Verification items for the finished model (mm, model axes). A direction names the side the tool comes from. Give positions to 0.01 mm unless a question says otherwise; leave off trailing zeros. Loops run counter-clockwise (first coordinate to the right, second up) from the corner with the lowest first, then second, coordinate; pieces in that order, holes last. Notation, with made-up numbers: (35.25, 86.5) -> (81.25, 86.5) arc R18 cw to (81.25, 92.5) -> close; hole circle Ø5 at (-7.5, -11). An arc over 180 degrees is marked (long way). Answer in a Markdown table with one row per item. Add a question column.
Q1. Gauge pin test, flat ends, axial feed: P1, Ø4, axis at x = 78.97, y = 68.18, coming from the +Z side; P2, Ø6, axis at y = 53, z = 3, coming from the +X side; P3, Ø6.5, axis at y = 95.5, z = 8, coming from the +X side; P4, Ø4, axis at x = 144, z = 3, coming from the -Y side. Record the tip position at first contact, or that the pin passes through.
Q2. Material ranges on probe 1 along Y at (x, z) = (88, 7.25); probe 2 along X at (y, z) = (67, 4.25); probe 3 along X at (y, z) = (43.5, 6), recorded low to high.
Q3. Section check B-B on z = 2.5. Give the number of separate pieces and of enclosed holes in the cut face, and give its area (3 significant figures).
Q4. Release check for a two-part mould opening along X. For faces 4 (the face through (6.16, 62, 6.41)), 5 (the face through (143.55, 20.69, 6.41)), 6 (the face through (38.49, 7.41, 6.41)) record: pulls with the +X half, pulls with the -X half, needs draft (parallel to the pull), parting line crosses it, or undercut.
Q5. Section check D-D on y = 36. Enter the section's corners in (x, z).
Q6. Section check A-A on y = 47. Enter the section's corners in (x, z).
Q7. Section check C-C on x = 153.5. Enter the section's corners in (y, z).
Q8. Set-up check for faces 1 (the face through (59.37, 14.43, 6.41)), 2 (the face through (128.62, 71.9, 6.41)), 3 (the face through (146.511, 82.857, 6.409)): record each of +Z, -Z, +X, -X, +Y, -Y from which the full face is reachable in a straight line by a thin tool's end or side.
```python
from build123d import *

# Parameters (mm, degrees)
ESBO_O1_R                = 3.175
RESSALTO_EXTRUS_O1_DEPTH = 13


with BuildPart() as part:
    # Esboço1 → Ressalto-extrusão1 (new body)
    with BuildSketch(Plane.XY):
        with BuildLine():
            Line((35.385230037, 10.075467345), (3.022965856, 59.821309359))
            Line((3.022965856, 59.821309359), (9.389592457, 64.241305524))
            ThreePointArc((9.389592457, 64.241305524), (12.424025355, 62.134521854), (16.11664555, 62.238812532))
            Line((16.11664555, 62.238812532), (37.995734983, 76.310625699))
            Line((37.995734983, 76.310625699), (73.510181395, 78.362700262))
            ThreePointArc((73.510181395, 78.362700262), (77.993066809, 80.699414035), (80.140456658, 85.276007717))
            Line((80.140456658, 85.276007717), (79.930003073, 94.415706286))
            Line((79.930003073, 94.415706286), (79.930003073, 97.029046835))
            ThreePointArc((79.930003073, 97.029046835), (101.572218687, 91.878964915), (121.946388489, 100.812163968))
            Line((121.946388489, 100.812163968), (121.946388489, 97.854479056))
            Line((121.946388489, 97.854479056), (121.946388489, 87.306940797))
            ThreePointArc((121.946388489, 87.306940797), (124.605004373, 83.87722317), (128.400566482, 81.773676237))
            Line((128.400566482, 81.773676237), (165.135958914, 83.971302002))
            Line((165.135958914, 83.971302002), (186.825026221, 73.136677472))
            ThreePointArc((186.825026221, 73.136677472), (191.417140339, 72.651683009), (195.305426608, 75.142458308))
            Line((195.305426608, 75.142458308), (201.904648359, 71.689614729))
            ThreePointArc((201.904648359, 71.689614729), (180.384547639, 42.366647273), (150.812504997, 21.190116644))
            ThreePointArc((150.812504997, 21.190116644), (150.313679981, 20.942400372), (149.813666262, 20.697092344))
            ThreePointArc((149.813666262, 20.697092344), (143.468376798, 20.722988132), (139.020600507, 25.248543905))
            ThreePointArc((139.020600507, 25.248543905), (106.562536674, 52.191838172), (72.546533139, 27.244322919))
            ThreePointArc((72.546533139, 27.244322919), (59.147798476, 14.281047119), (41.970794252, 7.033762392))
            ThreePointArc((41.970794252, 7.033762392), (38.439332559, 7.432489412), (35.662068876, 9.64992292))
            Line((35.662068876, 9.64992292), (35.385230037, 10.075467345))
        make_face()
        with Locations((89.421948725, 79.437523552)):
            Circle(ESBO_O1_R, mode=Mode.SUBTRACT)
        with Locations((113.572558486, 80.849829661)):
            Circle(ESBO_O1_R, mode=Mode.SUBTRACT)
        with Locations((78.965142383, 68.179773497)):
            Circle(ESBO_O1_R, mode=Mode.SUBTRACT)
        with Locations((125.590943677, 70.946640577)):
            Circle(ESBO_O1_R, mode=Mode.SUBTRACT)
    extrude(amount=RESSALTO_EXTRUS_O1_DEPTH)


solid = part.part
```
Taken from the geometry:
| question | item | result |
|---|---|---|
| 1 | P1 | passes through |
| 1 | P2 | stops at x = 192.18 |
| 1 | P3 | stops at x = 121.95 |
| 1 | P4 | stops at y = 20.1 |
| 2 | probe 1 | y = 47.38 to 76.6, 82.28 to 93.33 |
| 2 | probe 2 | x = 23.52 to 76.02, 81.91 to 199.35 |
| 2 | probe 3 | x = 13.64 to 82.71, 128.36 to 181.52 |
| 3 | separate pieces | 1 |
| 3 | enclosed holes | 4 |
| 3 | area | 8,820 mm² |
| 4 | face 4 | pulls with the -X half |
| 4 | face 5 | undercut |
| 4 | face 6 | parting line crosses it |
| 5 | outline | (18.52, 0) -> (76.41, 0) -> (76.41, 13) -> (18.52, 13) -> close; (134.66, 0) -> (173.39, 0) -> (173.39, 13) -> (134.66, 13) -> close |
| 6 | outline | (11.36, 0) -> (87.37, 0) -> (87.37, 13) -> (11.36, 13) -> close; (123.7, 0) -> (184.82, 0) -> (184.82, 13) -> (123.7, 13) -> close |
| 7 | outline | (22.58, 0) -> (83.28, 0) -> (83.28, 13) -> (22.58, 13) -> close |
| 8 | face 1 | +Z, -Z, -Y |
| 8 | face 2 | +Z, -Z |
| 8 | face 3 | +Z, -Z, +Y |
